Could you check a few things on this model? Use its own coordinates, in mm. A direction names the side the tool comes from. Coordinates: 2 decimals unless noted, no trailing zeros. Order: outer loops, then holes, each group sorted by start corner. A loop starts at its lowest first (then second) coordinate and runs counter-clockwise, first axis right, second up. Notation, with made-up numbers: (39, -37) - (62, -37) arc R12 ccw to (62, -17) - close; hole circle Ø2 at (57, 69). An arc over 180 degrees is marked (long way). One line per item, written item: value.
from build123d import *

# Parameters (mm, degrees)
SKETCH_R        = 4
PAD_DEPTH       = 100
SKETCH001_R     = 1
POCKET_DEPTH    = 5
SKETCH002_R     = 7
PAD001_DEPTH    = 20
SKETCH003_R     = 5.5
POCKET001_DEPTH = 15


with BuildPart() as part:
    # Sketch → Pad (new body)
    with BuildSketch(Plane.XY):
        Circle(SKETCH_R)
    extrude(amount=-PAD_DEPTH)

    # Sketch001 → Pocket (cut)
    with BuildSketch(Plane.XY):
        Circle(SKETCH001_R)
    extrude(amount=-POCKET_DEPTH, mode=Mode.SUBTRACT)

    # Sketch002 → Pad001 (new body)
    with BuildSketch(Plane(origin=(0, 0, -100), x_dir=(1, 0, 0), z_dir=(0, 0, -1))):
        Circle(SKETCH002_R)
    extrude(amount=PAD001_DEPTH)

    # Sketch003 → Pocket001 (cut)
    with BuildSketch(Plane(origin=(0, 0, -120), x_dir=(1, 0, 0), z_dir=(0, 0, -1))):
        Circle(SKETCH003_R)
    extrude(amount=-POCKET001_DEPTH, mode=Mode.SUBTRACT)


solid = part.part
Item 1: I want a section at A-A on y = 0. Please give me the cut outline in (x, z), then the cut area to 3 significant figures.
Conclusion:
outline: (-7, -120) - (-5.5, -120) - (-5.5, -105) - (5.5, -105) - (5.5, -120) - (7, -120) - (7, -100) - (4, -100) - (4, 0) - (1, 0) - (1, -5) - (-1, -5) - (-1, 0) - (-4, 0) - (-4, -100) - (-7, -100) - close
area: 905 mm²
Item 2: I want a section at C-C on z = -80. Please give me the cut outline in (x, y), then the cut area to 3 significant figures.
Conclusion:
outline: circle Ø8 at (0, 0)
area: 50.3 mm²
Item 3: For faces 1 (the face through (0, 0, -105)), 2 (the face through (-4, 4, -120)), 3 (the face through (-0.867, -3.905, -49.3)), which set-ups out of +Z, -Z, +X, -X, +Y, -Y let a thin tool reach every point of the face, with its end or its side?
Conclusion:
face 1: -Z
face 2: -Z, +X, -X, +Y, -Y
face 3: +Z
Item 4: I'm going to push flat-ended pins straight in: pin 1 Ø2 at (x, z) = (-1.5, -71.5) entering from +Y; pin 2 Ø2 at (y, z) = (4.5, -54) entering from +X; pin 3 Ø3 at (y, z) = (0, -91) entering from +X. Where does each tip first touch, or does it pass through?
Conclusion:
pin 1: y = 3.97
pin 2: x = 1.94
pin 3: x = 4
Item 5: Thinking about a two-plate mould opening in X: for faces 4 (the face through (1, -1, 0)), 5 (the face through (6.466, 2.681, -109.86)), 6 (the face through (-1.19, 5.37, -112.6)), which applies, pulls with the +X half, pulls with the -X half, needs draft (parallel to the pull), parting line crosses it, or undercut?
Conclusion:
face 4: needs draft
face 5: parting line crosses it
face 6: undercut
Item 6: If I drill on probe 1 along Y at (x, z) = (0, -3.65); probe 2 along Z at (x, y) = (-4.25, -1.5); probe 3 along Z at (x, y) = (0.5, 0), over which ranges is the centre line in solid material (lowest first)?
Conclusion:
probe 1: -4 to -1, 1 to 4
probe 2: -105 to -100
probe 3: -105 to -5
